```python
from build123d import *

# Parameters (mm, degrees)
BOSS_EXTRUDE1_DEPTH = 15
FILLET1_R           = 5
SKETCH2_R           = 2.75
CUT_EXTRUDE1_DEPTH  = 34.73143068
CUT_EXTRUDE2_DEPTH  = 34.731430775


# Read off the part's stored shape, not the designer's step: Mirror1
with BuildPart() as part:
    # Sketch1 → Boss-Extrude1 (new body)
    with BuildSketch(Plane(origin=(0, 0, 0), x_dir=(0, 0, -1), z_dir=(1, 0, 0))):
        with BuildLine():
            ThreePointArc((-20.976176963, 1), (-14.491376746, 15.198684154), (0, 21))
            Line((0, 21), (0, 16))
            ThreePointArc((0, 16), (-10.95445115, 11.66190379), (-15.968719423, 1))
            Line((-15.968719423, 1), (-20.976176963, 1))
        make_face()
        with BuildLine():
            Line((-24.976176963, 1), (-20.976176963, 1))
            ThreePointArc((-20.976176963, 1), (-20.84987969, 2.506494942), (-20.615528128, 4))
            Line((-20.615528128, 4), (-24.976176963, 4))
            Line((-24.976176963, 4), (-24.976176963, 1))
        make_face()
    extrude(amount=BOSS_EXTRUDE1_DEPTH)

    # Fillet1
    fillet1_edges = [part.edges().sort_by_distance(p)[0] for p in [
        (7.5, 4, 20.615528128),
    ]]
    fillet(fillet1_edges, radius=FILLET1_R)

    # Sketch2 → Cut-Extrude1 (cut, through all)
    with BuildSketch(Plane(origin=(0, 4, 0), x_dir=(1, 0, 0), z_dir=(0, 1, 0))):
        with Locations(Location((7.5, -21.226176963, 0), (0, 0, 146.334508492))):
            Circle(SKETCH2_R)
    extrude(amount=CUT_EXTRUDE1_DEPTH, mode=Mode.SUBTRACT)

    # Sketch2<3> → Cut-Extrude2 (cut, through all)
    with BuildSketch(Plane(origin=(0, 4, 0), x_dir=(1, 0, 0), z_dir=(0, 1, 0))):
        with BuildLine():
            ThreePointArc((5.975, -21.226176963), (7.5, -22.751176963), (9.025, -21.226176963))
            Line((9.025, -21.226176963), (5.975, -21.226176963))
        make_face()
        with BuildLine():
            Line((5.975, -21.226176963), (9.025, -21.226176963))
            ThreePointArc((9.025, -21.226176963), (7.5, -19.701176963), (5.975, -21.226176963))
        make_face()
    extrude(amount=-CUT_EXTRUDE2_DEPTH, mode=Mode.SUBTRACT)

    # Mirror1: part across plane


with BuildPart() as part_1:
    add(part.part)
    add(part.part.mirror(Plane.XY))


solid = part_1.part
```
The model under review builds one solid part; all positions refer to its coordinate system, in mm. A direction names the side the tool comes from. Give positions to 0.01 mm unless a question says otherwise; leave off trailing zeros. Loops run counter-clockwise (first coordinate to the right, second up) from the corner with the lowest first, then second, coordinate; pieces in that order, holes last. Notation, with made-up numbers: (27.25, -9.5) - (54.25, -9.5) arc R8 cw to (54.25, 1.5) - close; hole circle Ø6 at (7, 81). An arc over 180 degrees is marked (long way). Answer as a JSON object with one key per item and string values.
Q1. Add section C-C on z = -1. State the section outline as (x, y) points, plus the area to 3 significant figures.
Worked out:
{"outline": "(0, 15.97) - (15, 15.97) - (15, 20.98) - (0, 20.98) - close", "area": "75.1 mm^2"}
Q2. Add section B-B on x = 13. State the section outline as (y, z) points, plus the area to 3 significant figures.
Worked out:
{"outline": "(1, -24.98) - (4, -24.98) - (4, -24.39) arc R5 cw to (7.27, -19.7) arc R21 ccw to (7.27, 19.7) arc R5 cw to (4, 24.39) - (4, 24.98) - (1, 24.98) - (1, 15.97) arc R16 cw to (1, -15.97) - close", "area": "311 mm^2"}
Q3. Insertion check: pin 1 (8 mm diameter, centred on x = 5, y = 15, fed in from -Z); pin 2 (8 mm diameter, centred on x = 9.5, y = 15.5, fed in from +Z); pin 3 (4 mm diameter, centred on x = 9.5, y = 8, fed in from +Z); pin 4 (3 mm diameter, centred on y = 8.5, z = -17, fed in from -X). Each pin has a flat end and moves straight along its axis. Give the tip position at first contact, or say it passes through.
Worked out:
{"pin 1": "stops at z = -17.89", "pin 2": "stops at z = 17.57", "pin 3": "stops at z = 20.33", "pin 4": "stops at x = 0"}
Q4. Add section A-A on x = 7.5. Count the separate pieces of the cut face and the enclosed holes in it, plus the area to 3 significant figures.
Worked out:
{"separate pieces": "3", "enclosed holes": "0", "area": "272 mm^2"}
Q5. For faces 4 (the flat face through (7.17, 4, -19.58)), 5 (the flat face through (7.4, 1, -19.5)), list the 3-axis set-ups (+Z, -Z, +X, -X, +Y, -Y) from which the entire face can be reached by the end or side of a thin tool; tool diameter is ignored.
Worked out:
{"face 4": "+Y", "face 5": "+Z, -Z, +X, -X, -Y"}
Q6. To check wall thickness, follow line 1 along Z through (x, y) = (7.5, 2.4); line 2 along Z through (x, y) = (7.5, 3.3); line 3 along Z through (x, y) = (7.5, 7.9). State the ranges of each line that lie inside material, in increasing order.
Worked out:
{"line 1": "z = -24.98 to -22.75, -19.7 to -15.82, 15.82 to 19.7, 22.75 to 24.98", "line 2": "z = -24.98 to -22.75, -19.7 to -15.66, 15.66 to 19.7, 22.75 to 24.98", "line 3": "z = -18.48 to -13.91, 13.91 to 18.48"}
Q7. Add section D-D on y = 18. State the section outline as (x, z) points, plus the area to 4 significant figures.
Worked out:
{"outline": "(0, -10.82) - (15, -10.82) - (15, 10.82) - (0, 10.82) - close", "area": "324.5 mm^2"}
Q8. Mouldability with a two-part tool opening along Z and no side actions: class faces 1 (the flat face through (15, 17, 0)), 2 (the cylindrical face through (9.272, 4.014, -24.012)), 3 (the cylindrical face through (7.169, 2.521, -22.715)) as +Z half, -Z half, draft (parallel to the pull), parting line (faces both ways), or undercut.
Worked out:
{"face 1": "draft", "face 2": "-Z half", "face 3": "undercut"}
